```python
from build123d import *

# Parameters (mm, degrees)
SKETCH_1_W                  = 90
SKETCH_1_H                  = 35
EXTRUDE_1_DEPTH             = 5
SKETCH_2_R                  = 1
CUT_EXTRUDE_1_DEPTH         = 49.541219597
PATTERN_LINEAR_1_COUNT      = 2
PATTERN_LINEAR_1_PITCH      = 30
PATTERN_LINEAR_1_COUNT_DIR2 = 2
PATTERN_LINEAR_1_PITCH_DIR2 = 14
SKETCH_3_R                  = 1.75
CUT_EXTRUDE_2_DEPTH         = 49.541219597
PATTERN_LINEAR_2_COUNT      = 2
PATTERN_LINEAR_2_PITCH      = 20
SKETCH_6_R                  = 1.5
CUT_EXTRUDE_3_DEPTH         = 49.541219597
FILLET_1_R                  = 3
FILLET_2_R                  = 3
FILLET_3_R                  = 3
FILLET_4_R                  = 3
HOLE_WIZARD_M3_1_D          = 2.5


with BuildPart() as part:
    # 草图1 → 凸台-拉伸1 (new body)
    with BuildSketch(Plane(origin=(0, 0, 0), x_dir=(1, 0, 0), z_dir=(0, 1, 0))):
        Rectangle(SKETCH_1_W, SKETCH_1_H)
    extrude(amount=EXTRUDE_1_DEPTH)

    # 草图2 → 切除-拉伸1 (cut, through all)
    with BuildSketch(Plane(origin=(0, 5, 0), x_dir=(1, 0, 0), z_dir=(0, 1, 0))):
        with Locations(Location((35, 7.5, 0), (0, 0, 270))):
            Circle(SKETCH_2_R)
    cut_extrude_1 = extrude(amount=-CUT_EXTRUDE_1_DEPTH, mode=Mode.SUBTRACT)

    # 阵列(线性)1: Cut-Extrude 1 2 × 2
    with Locations(*[(-i * PATTERN_LINEAR_1_PITCH, 0, j * PATTERN_LINEAR_1_PITCH_DIR2) for i in range(PATTERN_LINEAR_1_COUNT) for j in range(PATTERN_LINEAR_1_COUNT_DIR2) if (i, j) != (0, 0)]):
        add(cut_extrude_1, mode=Mode.SUBTRACT)

    # 草图3 → 切除-拉伸2 (cut, through all)
    with BuildSketch(Plane(origin=(0, 5, 0), x_dir=(1, 0, 0), z_dir=(0, 1, 0))):
        with Locations(Location((-20, 12.7, 0), (0, 0, 270))):
            Circle(SKETCH_3_R)
    cut_extrude_2 = extrude(amount=-CUT_EXTRUDE_2_DEPTH, mode=Mode.SUBTRACT)

    # 阵列(线性)2: 切除-拉伸2 ×2
    with Locations(*[(-i * PATTERN_LINEAR_2_PITCH, 0, 0) for i in range(1, PATTERN_LINEAR_2_COUNT)]):
        add(cut_extrude_2, mode=Mode.SUBTRACT)

    # 草图6 → 切除-拉伸3 (cut, through all)
    with BuildSketch(Plane(origin=(0, 5, 0), x_dir=(1, 0, 0), z_dir=(0, 1, 0))):
        with Locations(Location((-30, 3.7, 0), (0, 0, 270))):
            Circle(SKETCH_6_R)
    extrude(amount=-CUT_EXTRUDE_3_DEPTH, mode=Mode.SUBTRACT)

    # 圆角1
    fillet_1_edges = [part.edges().sort_by_distance(p)[0] for p in [
        (-45, 2.5, 17.5),
    ]]
    fillet(fillet_1_edges, radius=FILLET_1_R)

    # 圆角2
    fillet_2_edges = [part.edges().sort_by_distance(p)[0] for p in [
        (-45, 2.5, -17.5),
    ]]
    fillet(fillet_2_edges, radius=FILLET_2_R)

    # 圆角3
    fillet_3_edges = [part.edges().sort_by_distance(p)[0] for p in [
        (45, 2.5, -17.5),
    ]]
    fillet(fillet_3_edges, radius=FILLET_3_R)

    # 圆角4
    fillet_4_edges = [part.edges().sort_by_distance(p)[0] for p in [
        (45, 2.5, 17.5),
    ]]
    fillet(fillet_4_edges, radius=FILLET_4_R)

    # M3 螺纹孔1 (through all)
    with Locations(Plane(origin=(0, 5, 0), x_dir=(1, 0, 0), z_dir=(0, 1, 0))):
        with Locations((5, 7.5), (5, -6.5), (35, 7.5), (35, -6.5)):
            Hole(HOLE_WIZARD_M3_1_D / 2)


solid = part.part
```
Model file for the job. Use its own axes, mm. Round coordinates to 2 decimals unless told otherwise and drop trailing zeros. Write each loop counter-clockwise with the first axis right and the second up, starting at its lowest first coordinate (ties: lowest second). Pieces come first, ordered by that corner, then holes. Notation, with made-up numbers: (9, 75) - (20, 75) arc R17 ccw to (20, 90) - close; hole circle Ø4 at (69, 61.5). An arc over 180 degrees is marked (long way). One line per item, written item: value.
(1) Cut at C-C, the plane z = -3.7. Give the cut face in (x, y), plus the area to 3 significant figures.
Values follow:
outline: (-45, 0) - (-31.5, 0) - (-31.5, 5) - (-45, 5) - close; (-28.5, 0) - (45, 0) - (45, 5) - (-28.5, 5) - close
area: 435 mm²
(2) Cut at A-A, the plane y = 2.75. Give the cut face in (x, z).
Values follow:
outline: (-45, -14.5) arc R3 ccw to (-42, -17.5) - (42, -17.5) arc R3 ccw to (45, -14.5) - (45, 14.5) arc R3 ccw to (42, 17.5) - (-42, 17.5) arc R3 ccw to (-45, 14.5) - close; hole circle Ø3.5 at (-40, -12.7); hole circle Ø3 at (-30, -3.7); hole circle Ø3.5 at (-20, -12.7); hole circle Ø2.5 at (5, -7.5); hole circle Ø2.5 at (5, 6.5); hole circle Ø2.5 at (35, -7.5); hole circle Ø2.5 at (35, 6.5)
(3) Cut at D-D, the plane z = -7.5. Give the cut face in (x, y).
Values follow:
outline: (-45, 0) - (3.75, 0) - (3.75, 5) - (-45, 5) - close; (6.25, 0) - (33.75, 0) - (33.75, 5) - (6.25, 5) - close; (36.25, 0) - (45, 0) - (45, 5) - (36.25, 5) - close
(4) Wall check: probe 1 along X at (y, z) = (3.8, -7.5); probe 2 along Z at (x, y) = (35, 3.05); probe 3 along X at (y, z) = (2.1, -3.7). Give the ranges that are in metal, low to high.
Values follow:
probe 1: x = -45 to 3.75, 6.25 to 33.75, 36.25 to 45
probe 2: z = -17.5 to -8.75, -6.25 to 5.25, 7.75 to 17.5
probe 3: x = -45 to -31.5, -28.5 to 45
(5) Two-plate mould, pull along X, no slides. Class faces 1 (the flat face through (45, 2, 0)), 2 (the cylindrical face through (-18.265, 2.535, -12.928)), 3 (the flat face through (-1, 2, 17.5)), 4 (the cylindrical face through (-44.14, 2.54, 16.6)): pulls with the +X half, pulls with the -X half, needs draft (parallel to the pull), parting line crosses it, or undercut.
Values follow:
face 1: pulls with the +X half
face 2: undercut
face 3: needs draft
face 4: pulls with the -X half
(6) Cut at B-B, the plane x = 5. Give the cut face in (y, z), plus the area to 3 significant figures.
Values follow:
outline: (0, -17.5) - (5, -17.5) - (5, -8.75) - (0, -8.75) - close; (0, -6.25) - (5, -6.25) - (5, 5.25) - (0, 5.25) - close; (0, 7.75) - (5, 7.75) - (5, 17.5) - (0, 17.5) - close
area: 150 mm²
(7) Drop a flat-ended pin along its axis: P1, Ø4, axis at x = 5, z = 6.5, coming from the -Y side. Give the stop position or say it passes through.
Values follow:
P1: stops at y = 0
